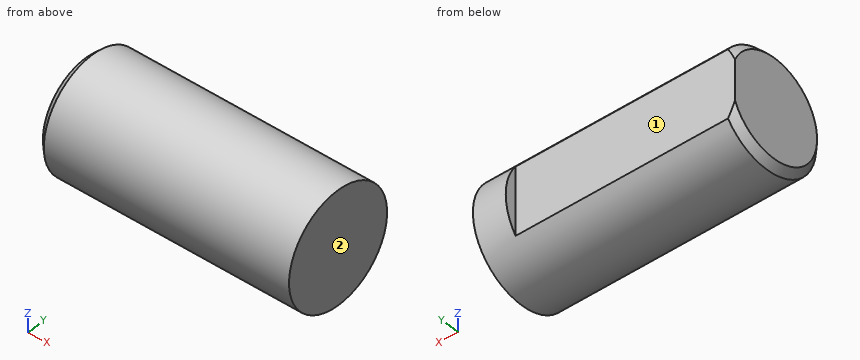
```python
from build123d import *

# Parameters (mm, degrees)
ESQUISSE1_W                  = 18
ESQUISSE1_H                  = 4
CHANFREIN1_SIZE              = 0.5
ENL_V_MAT_EXTRU_1_DEPTH      = 19.867962264
ENL_V_MAT_EXTRU_1_DEPTH_BACK = 19.867962264
ESQUISSE2_W                  = 17.317421693
ESQUISSE2_H                  = 9.702668892


with BuildPart() as part:
    # Esquisse1 → Base-Révolution (revolve)
    with BuildSketch(Plane.XY, mode=Mode.PRIVATE) as base_r_volution_sk:
        with Locations((-9, 2)):
            Rectangle(ESQUISSE1_W, ESQUISSE1_H)
    revolve(base_r_volution_sk.sketch.rotate(Axis((0, 0, 0), (-1, 0, 0)), 90), axis=Axis((0, 0, 0), (-1, 0, 0)))

    # Chanfrein1
    chanfrein1_edges = [part.edges().sort_by_distance(p)[0] for p in [
        (-18, 0, 4),
    ]]
    chamfer(chanfrein1_edges, length=CHANFREIN1_SIZE)

    # Esquisse2 → Enlèv. mat.-Extru.1 (cut, two sides: drawn at the far end of the back side and taken through both)
    with BuildSketch(Plane.XY.offset(-ENL_V_MAT_EXTRU_1_DEPTH_BACK)):
        with Locations((-11.002531853, 8.051334446)):
            Rectangle(ESQUISSE2_W, ESQUISSE2_H)
    extrude(amount=ENL_V_MAT_EXTRU_1_DEPTH + ENL_V_MAT_EXTRU_1_DEPTH_BACK, mode=Mode.SUBTRACT)


solid = part.part
```
For this review, take the finished solid that the model builds, in its own axes (mm). Face numbers are marked on the shaded views. A direction names the side the tool comes from. Give positions to 0.01 mm unless a question says otherwise; leave off trailing zeros. Order: outer loops, then holes, each group sorted by start corner. A loop starts at its lowest first (then second) coordinate and runs counter-clockwise, first axis right, second up.
1) Insertion check: pin 1 (2 mm diameter, centred on x = -12.5, y = -1, fed in from +Z); pin 2 (3 mm diameter, centred on x = -3.5, z = 2, fed in from -Y). Each pin has a flat end and moves straight along its axis. Give the tip position at first contact, or say it passes through.
2) Wall thickness on line 1 (Y direction, x = -11, z = 0); line 2 (Y direction, x = -13.25, z = -2); line 3 (Z direction, x = -10, y = -1.75): over which ranges is each line inside the solid? List them lowest first.
3) Take a section at B-B (x = -1.75). Give the boundary of the cut face in (y, z).
4) Take a section at A-A (z = 0). Give the boundary of the cut face in (x, y), then the cut area to 3 significant figures.
5) For the marked faces 1 and 2, list the 3-axis set-ups (+Z, -Z, +X, -X, +Y, -Y) from which the entire face can be reached by the end or side of a thin tool; tool diameter is ignored.
Derived:
1. pin 1: stops at z = 4
1. pin 2: stops at y = -3.97
2. line 1: y = -4 to 3.2
2. line 2: y = -3.46 to 3.2
2. line 3: z = -3.6 to 3.6
3. outline: circle Ø8 at (0, 0)
4. outline: (-18, -3.5) - (-17.5, -4) - (0, -4) - (0, 4) - (-2.34, 4) - (-2.34, 3.2) - (-18, 3.2) - close
4. area: 131 mm2
5. face 1: +Z, -Z, -X, +Y
5. face 2: +Z, -Z, +X, +Y, -Y
